```python
from build123d import *

# Parameters (mm, degrees)
SKETCH_1_R          = 1.6
EXTRUDE_1_DEPTH     = 2
CUT_EXTRUDE_1_DEPTH = 10
FILLET_1_R          = 5
FILLET_2_R          = 1.5


with BuildPart() as part:
    # ｽｹｯﾁ1 → ﾎﾞｽ - 押し出し1 (new body)
    with BuildSketch(Plane.XY):
        Polygon((-10.703193979, 31.538475775), (-21.961524228, 25.038475775), (-21.961524228, -25.038475775), (-10.703193979, -31.538475775), (32.664718207, -6.5), (32.664718207, 6.5), align=None)
        with Locations((-13.30127019, 23.038475775)):
            Circle(SKETCH_1_R, mode=Mode.SUBTRACT)
        with Locations((-13.30127019, -23.038475775)):
            Circle(SKETCH_1_R, mode=Mode.SUBTRACT)
        with Locations((26.602540381, 0)):
            Circle(SKETCH_1_R, mode=Mode.SUBTRACT)
    extrude(amount=EXTRUDE_1_DEPTH)

    # ｽｹｯﾁ2 → ｶｯﾄ - 押し出し1 (cut)
    with BuildSketch(Plane.XY.offset(2)):
        Polygon((-4.330127019, 0), (-14.461524228, 17.548094718), (-14.461524228, -17.548094718), align=None)
        Polygon((2.165063509, -3.75), (-7.9663337, -21.298094718), (22.427857928, -3.75), align=None)
        Polygon((22.427857928, 3.75), (-7.9663337, 21.298094718), (2.165063509, 3.75), align=None)
    extrude(amount=-CUT_EXTRUDE_1_DEPTH, mode=Mode.SUBTRACT)

    # ﾌｨﾚｯﾄ1
    fillet_1_edges = [part.edges().sort_by_distance(p)[0] for p in [
        (32.664718207, 6.5, 1),
        (32.664718207, -6.5, 1),
        (-10.703193979, -31.538475775, 1),
        (-21.961524228, -25.038475775, 1),
        (-21.961524228, 25.038475775, 1),
        (-10.703193979, 31.538475775, 1),
        (-4.330127019, 0, 1),
        (2.165063509, -3.75, 1),
        (2.165063509, 3.75, 1),
    ]]
    fillet(fillet_1_edges, radius=FILLET_1_R)

    # ﾌｨﾚｯﾄ2
    fillet_2_edges = [part.edges().sort_by_distance(p)[0] for p in [
        (-14.461524228, 17.548094718, 1),
        (-14.461524228, -17.548094718, 1),
        (22.427857928, -3.75, 1),
        (-7.9663337, -21.298094718, 1),
        (-7.9663337, 21.298094718, 1),
        (22.427857928, 3.75, 1),
    ]]
    fillet(fillet_2_edges, radius=FILLET_2_R)


solid = part.part
```
Verification items for the finished model (mm, model axes). A direction names the side the tool comes from. Coordinates: 2 decimals unless noted, no trailing zeros. Write each loop counter-clockwise with the first axis right and the second up, starting at its lowest first coordinate (ties: lowest second). Pieces come first, ordered by that corner, then holes. Notation, with made-up numbers: M -36,-31.75 L 7,-31.75 A22 ccw 7,-5.75 Z; hole C 77,71.25 d7. An arc over 180 degrees is marked long. Answer as a JSON object with one key per item and string values. Group by question number.
(1) Material ranges on line 1 (Y direction, x = 7, z = 0.9); line 2 (Y direction, x = 2, z = 0.45); line 3 (X direction, y = 8.5, z = 1.4), recorded low to high.
(2) Cross-section at B-B, the plane z = 1.5. State how many separate pieces and enclosed holes the cut face has, and give its area (3 significant figures).
(3) Release check for a two-part mould opening along X. For faces 3 (the face through (-10.74, 30.765, 1.014)), 4 (the face through (-4.95, 18.24, 0.99)), 5 (the face through (32.665, 0, 1)), 6 (the face through (-11.823, -23.651, 0.986)) record: +X half, -X half, draft (parallel to the pull), parting line (faces both ways), or undercut.
(4) Cross-section at A-A, the plane y = 0. Record the cut outline in (x, z).
(5) Cross-section at D-D, the plane x = 20. Record the cut outline in (y, z).
(6) Cross-section at C-C, the plane x = 2. Record the cut outline in (y, z).
(7) Tool access check on faces 1 (the face through (7.1, -12.6, 1)), 2 (the face through (32.013, -6.081, 1.014)). Record the directions out of +Z, -Z, +X, -X, +Y, -Y that give a thin tool (end or side, any length) a straight path to the whole face; none if there is none.
(8) Gauge pin test, flat ends, axial feed: pin 1 (0.6 mm diameter, centred on x = 13, z = 0.5, fed in from +Y); pin 2 (1 mm diameter, centred on x = 2.5, z = 1.5, fed in from +Y). Record the tip position at first contact, or that the pin passes through.
Reply:
{
 "1": {"line 1": "-21.32 to -12.66, -3.75 to 3.75, 12.66 to 21.32", "line 2": "-24.2 to -15.54, -4.79 to 4.79, 15.54 to 24.2", "line 3": "-21.96 to -14.46, -9.24 to -0.58, 14.2 to 29.2"},
 "2": {"separate pieces": "1", "enclosed holes": "6", "area": "1,760 mm²"},
 "3": {"face 3": "parting line", "face 4": "undercut", "face 5": "+X half", "face 6": "undercut"},
 "4": {"outline": "M -21.96,0 L -14.46,0 L -14.46,2 L -21.96,2 Z; M -5.1,0 L 25,0 L 25,2 L -5.1,2 Z; M 28.2,0 L 32.66,0 L 32.66,2 L 28.2,2 Z"},
 "5": {"outline": "M -13.81,0 L 13.81,0 L 13.81,2 L -13.81,2 Z"},
 "6": {"outline": "M -24.2,0 L -15.54,0 L -15.54,2 L -24.2,2 Z; M -4.79,0 L 4.79,0 L 4.79,2 L -4.79,2 Z; M 15.54,0 L 24.2,0 L 24.2,2 L 15.54,2 Z"},
 "7": {"face 1": "+Z, -Z", "face 2": "+Z, -Z, +X, -Y"},
 "8": {"pin 1": "y = 18.03", "pin 2": "y = 24.2"}
}
